Autodesk Inventor part; units mm, degrees
ref_plane "YZ Plane" through (0, 0, 0) normal (1, 0, 0) x (0, 1, 0)
ref_plane "XZ Plane" through (0, 0, 0) normal (0, 1, 0) x (-1, 0, 0)
ref_plane "XY Plane" through (0, 0, 0) normal (0, 0, 1) x (1, 0, 0)
ref_plane "작업 평면1" through (0, 0, 0) normal (0, 0, 1) x (1, 0, 0)
sketch "스케치1" plane through (0, 0, 0) normal (0, 0, 1) x (1, 0, 0)
  circle A0 centre (28.8901, -8.5) radius 5
  circle A1 centre (28.8901, -8.5) radius 5.3
  circle A2 centre (28.8901, -8.5) radius 7
  line L0 (46.6099, 5.5) -> (-13.1099, 5.5)
  line L1 (46.6099, -16.5) -> (46.6099, 5.5)
  line L2 (35.8901, -8.5) -> (35.8901, 5.5)
  line L3 (21.8901, -8.5) -> (21.8901, 5.5)
  line L4 (35.8901, 5.5) -> (21.8901, 5.5)
  line L5 (21.8901, 5.5) -> (21.8901, 8.7184)
  line L6 (21.8901, 8.7184) -> (35.8901, 8.7184)
  line L7 (35.8901, 8.7184) -> (35.8901, 5.5)
  line L8 (21.8901, 5.5) -> (35.8901, 5.5)
  point P0 (0, 0)
  point P1 (21.8901, 5.5)
  dimension "d0" = 0.3
  dimension "d1" = 2
extrude "돌출1" add sketch "스케치1" along normal blind 2 contours A2 | A2 L3 L0 L2 | L0 L5 L6 L7
sketch "스케치2" plane through (0, 0, 0) normal (0, 0, -1) x (-1, 0, 0)
  line L0 (-21.8901, 8.7184) -> (-21.8901, -8.5)
  line L1 (-35.8901, 8.7184) -> (-21.8901, 8.7184)
  line L2 (-35.8901, -8.5) -> (-35.8901, 8.7184)
  line L3 (13.1099, 5.5) -> (-46.6099, 5.5)
  point P0 (0, 0)
  point P1 (-35.8901, 5.5)
  point P2 (-21.8901, 5.5)
extrude "돌출2" add sketch "스케치2" against normal blind 25
properties material "고무, 검은색"
Geometry: final body of the model. Coordinates: model frame, mm. A direction names the side the tool comes from. Round coordinates to 2 decimals unless told otherwise and drop trailing zeros. Write each loop counter-clockwise with the first axis right and the second up, starting at its lowest first coordinate (ties: lowest second). Pieces come first, ordered by that corner, then holes. Notation, with made-up numbers: (-37, -29.75) -> (-7, -29.75) arc R17 ccw to (-7, -8.75) -> close; hole circle Ø11 at (-5, -24.5). An arc over 180 degrees is marked (long way). Use CSV: the item, a comma, the result in double quotes. Start each with the question number.
Q1. First-contact query: pin 1 Ø3 at (x, y) = (32, -10.5) entering from +Z; pin 2 Ø2 at (x, y) = (31.5, -1) entering from +Z; pin 3 Ø5 at (x, z) = (28.5, 10) entering from -Y. Flat tips, straight axial feed; report the tip coordinate or a pass-through.
Q2. Section A-A (x = 29.5). Return loops of the section in (y, z), plus the area to 3 significant figures.
Q3. Reachability of faces 4 (the face through (29, -15.5, 1)), 5 (the face through (29, -3, 2)) from +Z, -Z, +X, -X, +Y, -Y: full face, straight path, thin tool, end or side. Return the list, or none.
Q4. Section B-B (y = -4). Return loops of the section in (x, z), plus the area to 3 significant figures.
Q5. Pull-direction query (X, two-part tool) for faces 1 (the face through (21.89, 6, 10)), 2 (the face through (29, 7, 25)), 3 (the face through (24.68, -5.28, 0.99)); classes: pulls with the +X half, pulls with the -X half, needs draft (parallel to the pull), parting line crosses it, or undercut.
Q6. Line query: L1, parallel to Z at x = 24.5, y = 5.25; L2, parallel to Y at x = 29.5, z = 11.75. Output: solid intervals per line, ascending.
Q7. Section C-C (x = 34.5). Return loops of the section in (y, z).
Q8. Section D-D (z = 9). Return loops of the section in (x, y), plus the area to 3 significant figures.
Result sheet:
1,pin 1,"through"
1,pin 2,"z = 2"
1,pin 3,"y = 5.5"
2,outline,"(-15.47, 0) -> (-13.76, 0) -> (-13.76, 2) -> (-15.47, 2) -> close; (-3.24, 0) -> (8.72, 0) -> (8.72, 25) -> (5.5, 25) -> (5.5, 2) -> (-3.24, 2) -> close"
2,area,"101 mm²"
3,face 4,"+Z, -Z, -Y"
3,face 5,"+Z, +X, -X, -Y"
4,outline,"(21.89, 0) -> (26.09, 0) -> (26.09, 2) -> (21.89, 2) -> close; (31.69, 0) -> (35.89, 0) -> (35.89, 2) -> (31.69, 2) -> close"
4,area,"16.8 mm²"
5,face 1,"pulls with the -X half"
5,face 2,"needs draft"
5,face 3,"undercut"
6,L1,"0 to 2"
6,L2,"5.5 to 8.72"
7,outline,"(-12.69, 0) -> (8.72, 0) -> (8.72, 25) -> (5.5, 25) -> (5.5, 2) -> (-12.69, 2) -> close"
8,outline,"(21.89, 5.5) -> (35.89, 5.5) -> (35.89, 8.72) -> (21.89, 8.72) -> close"
8,area,"45.1 mm²"
